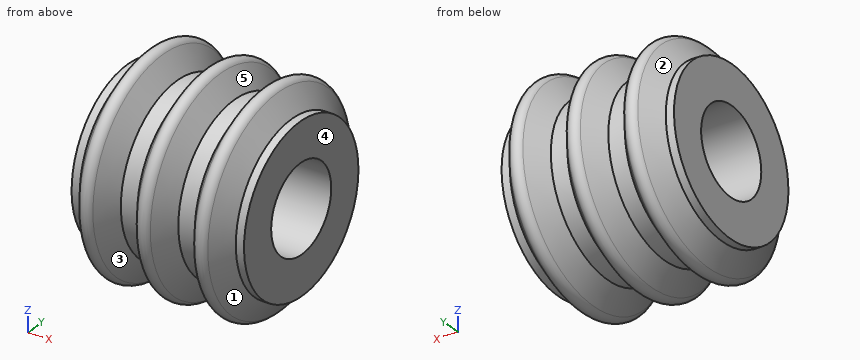
```python
from build123d import *

# Parameters (mm, degrees)
F2_R     = 5.254137
F3_DEPTH = 21.001


with BuildPart() as f1:
    # F0 (on Front) → F1 (revolve)
    with BuildSketch(Plane.XZ):
        with BuildLine():
            Line((-10.5, 35.596944), (-10.5, 25.596944))
            Line((-10.5, 25.596944), (10.5, 25.596944))
            Line((10.5, 25.596944), (10.5, 35.596944))
            Line((10.5, 35.596944), (9.5, 35.596944))
            Line((9.5, 35.596944), (7.831313, 38.092791))
            ThreePointArc((7.831313, 38.092791), (7, 38.536987), (6.168687, 38.092791))
            Line((6.168687, 38.092791), (4.5, 35.596944))
            Line((4.5, 35.596944), (2.5, 35.596944))
            Line((2.5, 35.596944), (0.831313, 38.092791))
            ThreePointArc((0.831313, 38.092791), (0, 38.536987), (-0.831313, 38.092791))
            Line((-0.831313, 38.092791), (-2.5, 35.596944))
            Line((-2.5, 35.596944), (-4.5, 35.596944))
            Line((-4.5, 35.596944), (-6.168687, 38.092791))
            ThreePointArc((-6.168687, 38.092791), (-7, 38.536987), (-7.831313, 38.092791))
            Line((-7.831313, 38.092791), (-9.5, 35.596944))
            Line((-9.5, 35.596944), (-10.5, 35.596944))
        make_face()
    revolve(axis=Axis((0, 0, 25.596944), (1, 0, 0)))

    # F2 (on face) → F3 (cut, through all)
    with BuildSketch(Plane(origin=(-10.5, 0, 0), x_dir=(0, -1, 0), z_dir=(-1, 0, 0))):
        with Locations((0, 25.596944)):
            Circle(F2_R)
    extrude(amount=-F3_DEPTH, mode=Mode.SUBTRACT)


solid = f1.part
```
Read the model definition and answer for the solid it produces. Units are mm, in the model's axes. Face numbers are marked on the shaded views. A direction names the side the tool comes from. Round coordinates to 2 decimals unless told otherwise and drop trailing zeros. Write each loop counter-clockwise with the first axis right and the second up, starting at its lowest first coordinate (ties: lowest second). Pieces come first, ordered by that corner, then holes. Notation, with made-up numbers: M -9,55 L 22,55 A25 ccw 22,93 Z; hole C -35.75,25 d9. An arc over 180 degrees is marked long. One line per item, written item: value.
Q1. For a pull along X with two mould halves and no side action, classify the marked faces 1, 2 and 3 as +X half, -X half, draft (parallel to the pull), parting line (faces both ways), or undercut.
Data:
face 1: +X half
face 2: -X half
face 3: undercut
Q2. Straight lines are drawn through the part: line 1 (X direction, y = -5.75, z = 15.5); line 2 (Z direction, x = -4.25, y = 0); line 3 (X direction, y = 4, z = 35.5). For each, find the intervals that lie inside material, in ascending order. Write a range as [from, to].
Data:
line 1: [-8.42, -5.58], [-1.42, 1.42], [5.58, 8.42]
line 2: [15.6, 20.34], [30.85, 35.6]
line 3: [-9.05, -4.95], [-2.05, 2.05], [4.95, 9.05]
Q3. Flat-ended cylindrical pins translate along their axes: pin 1 Ø6 at (x, z) = (6, 27.5) entering from +Y; pin 2 Ø1.5 at (x, z) = (-1, 29.5) entering from -Y; pin 3 Ø5 at (x, z) = (-1, 21.5) entering from -Y; pin 4 Ø12 at (x, y) = (-6, -7) entering from +Z. Find the tip coordinate at first contact, or state that the pin passes through.
Data:
pin 1: y = 12.94
pin 2: y = -12.39
pin 3: y = -12.82
pin 4: z = 38.49
Q4. Find section B-B on x = 5. Write down the section's boundary in (y, z), plus the area to 3 significant figures.
Data:
outline: C 0,25.6 d21.5; hole C 0,25.6 d10.51
area: 276 mm2
Q5. Find section C-C on z = 36.5. Count the separate pieces of the cut face and the enclosed holes in it, plus the area to 3 significant figures.
Data:
separate pieces: 3
enclosed holes: 0
area: 118 mm2
Q6. Which of the six approach directions +Z, -Z, +X, -X, +Y, -Y give full straight-line access (tool end or side, diameter ignored) to the marked faces 4 and 5?
Data:
face 4: +Z, -Z, +X, +Y, -Y
face 5: none
